Source: CAD feature listing. Evaluate the final solid. Frame: model axes, mm. A direction names the side the tool comes from. Give positions to 0.01 mm unless a question says otherwise; leave off trailing zeros. Loops run counter-clockwise (first coordinate to the right, second up) from the corner with the lowest first, then second, coordinate; pieces in that order, holes last. Notation, with made-up numbers: (89.5, -33) - (117.5, -33) arc R29 ccw to (117.5, -3) - close; hole circle Ø2 at (38, 1.5). An arc over 180 degrees is marked (long way). Put each result on its own line as item: value.
```python
from build123d import *

# Parameters (mm, degrees)
SKETCH1_R                = 18.5
BOSS_EXTRUDE1_DEPTH      = 1.5
SKETCH2_R                = 18.5
SKETCH2_R_2              = 17
BOSS_EXTRUDE2_DEPTH      = 5
SKETCH3_W                = 13
SKETCH3_H                = 71.108724116
BOSS_EXTRUDE3_DEPTH      = 0.5
BOSS_EXTRUDE3_DEPTH_BACK = 1.5
SKETCH4_R                = 3
BOSS_EXTRUDE4_DEPTH      = 2
BOSS_EXTRUDE4_DEPTH_BACK = 0.5
CUT_EXTRUDE1_DEPTH       = 2
SKETCH7_R                = 1.4
CUT_EXTRUDE2_DEPTH       = 3


with BuildPart() as part:
    # Sketch1 → Boss-Extrude1 (new body)
    with BuildSketch(Plane(origin=(0, 0, 0), x_dir=(1, 0, 0), z_dir=(0, 1, 0))):
        Circle(SKETCH1_R)
    extrude(amount=BOSS_EXTRUDE1_DEPTH)

    # Sketch2 → Boss-Extrude2 (add)
    with BuildSketch(Plane(origin=(0, 1.5, 0), x_dir=(1, 0, 0), z_dir=(0, 1, 0))):
        Circle(SKETCH2_R)
        Circle(SKETCH2_R_2, mode=Mode.SUBTRACT)
    extrude(amount=BOSS_EXTRUDE2_DEPTH)

    # Sketch3 → Boss-Extrude3 (add, two sides)
    with BuildSketch(Plane(origin=(0, 0, 0), x_dir=(-1, 0, 0), z_dir=(0, -1, 0))) as boss_extrude3_sk:
        with Locations((0, 24.445637942)):
            Rectangle(SKETCH3_W, SKETCH3_H)
    extrude(amount=BOSS_EXTRUDE3_DEPTH)
    extrude(boss_extrude3_sk.sketch, amount=-BOSS_EXTRUDE3_DEPTH_BACK)

    # Sketch4 → Boss-Extrude4 (add, two sides)
    with BuildSketch(Plane(origin=(0, -0.5, 0), x_dir=(-1, 0, 0), z_dir=(0, -1, 0))) as boss_extrude4_sk:
        with Locations((3.5, -9.108724116)):
            Circle(SKETCH4_R)
        with Locations((-3.5, 49.5)):
            Circle(SKETCH4_R)
        with Locations((-3.5, -9.108724116)):
            Circle(SKETCH4_R)
    extrude(amount=BOSS_EXTRUDE4_DEPTH)
    extrude(boss_extrude4_sk.sketch, amount=-BOSS_EXTRUDE4_DEPTH_BACK)

    # Sketch6 → Cut-Extrude1 (cut)
    with BuildSketch(Plane(origin=(0, -2.5, 0), x_dir=(-1, 0, 0), z_dir=(0, -1, 0))):
        with BuildLine():
            Line((-3.5, 51.5), (-3.5, 52.5))
            ThreePointArc((-3.5, 52.5), (-0.5, 49.5), (-3.5, 46.5))
            Line((-3.5, 46.5), (-3.5, 47.5))
            ThreePointArc((-3.5, 47.5), (-1.5, 49.5), (-3.5, 51.5))
        make_face()
    extrude(amount=-CUT_EXTRUDE1_DEPTH, mode=Mode.SUBTRACT)

    # Sketch7 → Cut-Extrude2 (cut)
    with BuildSketch(Plane(origin=(0, -2.5, 0), x_dir=(-1, 0, 0), z_dir=(0, -1, 0))):
        with Locations((-3.5, 49.5)):
            Circle(SKETCH7_R)
        with Locations((3.5, -9.108724116)):
            Circle(SKETCH7_R)
    extrude(amount=-CUT_EXTRUDE2_DEPTH, mode=Mode.SUBTRACT)


solid = part.part
```
1) Section query B-B, the plane y = 4.25. Output: boundary loops of the cut face in (x, z).
Check result:
outline: circle Ø37 at (0, 0); hole circle Ø34 at (0, 0)
2) Mould query, pull axis X, two halves, no side actions, for faces 4 (the cylindrical face through (1.5, -1.5, -49.5)), 5 (the flat face through (0, 1.5, 0)), 6 (the cylindrical face through (8.54, 3.2, 16.41)), 7 (the flat face through (0, 1.5, -39)). Classes: pulls with the +X half, pulls with the -X half, needs draft (parallel to the pull), parting line crosses it, or undercut.
Check result:
face 4: pulls with the -X half
face 5: undercut
face 6: parting line crosses it
face 7: needs draft
3) Section query A-A, the plane x = 9.5. Output: boundary loops of the cut face in (y, z), plus the area to 3 significant figures.
Check result:
outline: (0, -15.87) - (6.5, -15.87) - (6.5, -14.1) - (1.5, -14.1) - (1.5, 14.1) - (6.5, 14.1) - (6.5, 15.87) - (0, 15.87) - close
area: 65.4 mm²
4) Access query for faces 1 (the cylindrical face through (9.139, 3.965, -14.334)), 2 (the cylindrical face through (6.5, -1.5, -49.6)), 3 (the cylindrical face through (-4.793, -1.021, 9.645)). Directions: +Z, -Z, +X, -X, +Y, -Y. A direction counts if a zero-diameter tool reaches every point of the face in a straight line with its end or side. Return the directions, or none.
Check result:
face 1: +Y
face 2: +X, -Y
face 3: -Y
5) Section query D-D, the plane x = -7.5. Output: boundary loops of the cut face in (y, z), plus the area to 3 significant figures.
Check result:
outline: (0, -16.91) - (6.5, -16.91) - (6.5, -15.26) - (1.5, -15.26) - (1.5, 15.26) - (6.5, 15.26) - (6.5, 16.91) - (0, 16.91) - close
area: 67.3 mm²
6) Material intervals for line 1 along Z through (x, y) = (0, 2.9); line 2 along Z through (x, y) = (3.5, -0.15); line 3 along Y through (x, z) = (-0.5, -5), sorted ascending. Write a range as [from, to].
Check result:
line 1: [-18.5, -17], [17, 18.5]
line 2: [-60, -50.9], [-48.1, 12.11]
line 3: [-0.5, 1.5]
7) Section query C-C, the plane z = 0. Output: boundary loops of the cut face in (x, y), plus the area to 3 significant figures.
Check result:
outline: (-18.5, 0) - (-6.5, 0) - (-6.5, -0.5) - (6.5, -0.5) - (6.5, 0) - (18.5, 0) - (18.5, 6.5) - (17, 6.5) - (17, 1.5) - (-17, 1.5) - (-17, 6.5) - (-18.5, 6.5) - close
area: 77.0 mm²
8) Pin query (flat end, axial travel): P1, Ø4, axis at y = 3, z = -49.5, coming from the +X side; P2, Ø3, axis at x = 10, z = -9, coming from the -Y side; P3, Ø5, axis at x = 8.5, y = 0.5, coming from the +Z side. Return the tip coordinate at first contact, or that it passes through.
Check result:
P1: x = 6.5
P2: y = 0
P3: z = 17.5
